Source: CAD feature listing. Evaluate the final solid. Frame: model axes, mm. Give positions to 0.01 mm unless a question says otherwise; leave off trailing zeros. Loops run counter-clockwise (first coordinate to the right, second up) from the corner with the lowest first, then second, coordinate; pieces in that order, holes last. Notation, with made-up numbers: M 4,65.5 L 27,65.5 A21 cw 27,91.5 Z; hole C 5.25,-28.75 d4. An arc over 180 degrees is marked long. Write item = value, one per line.
from build123d import *

# Parameters (mm, degrees)
F0_R     = 2.5
F1_DEPTH = 4.85
F4_DEPTH = 3
F6_DEPTH = 5


with BuildPart() as f1:
    # F0 (on Front) → F1 (new body)
    with BuildSketch(Plane.XZ):
        with BuildLine():
            Line((0, 10.100125), (0, 5))
            Line((0, 5), (-2, 5))
            Line((-2, 5), (-2, -5))
            Line((-2, -5), (0, -5))
            Line((0, -5), (0, -9.588868))
            ThreePointArc((0, -9.588868), (0.776393, -10.563548), (1.9, -10.024758))
            Line((1.9, -10.024758), (1.9, -9.493749))
            Line((1.9, -9.493749), (101.874922, -4.488743))
            Line((101.874922, -4.488743), (106.868668, -4.238743))
            ThreePointArc((106.868668, -4.238743), (111.143668, 0.255629), (106.868668, 4.75))
            Line((106.868668, 4.75), (101.874922, 5))
            Line((101.874922, 5), (1.9, 10.005006))
            Line((1.9, 10.005006), (1.9, 10.71228))
            ThreePointArc((1.9, 10.71228), (0.845568, 11.433139), (0, 10.47581))
            Line((0, 10.47581), (0, 10.100125))
        make_face()
        Polygon((13.94009, -6.988611), (1.9, -7.59137), (1.9, 0.047531), (1.9, 6.476616), align=None, mode=Mode.SUBTRACT)
        Polygon((40.412243, -5.663346), (16.82521, -6.844175), (30.799962, 5.351317), align=None, mode=Mode.SUBTRACT)
        Polygon((43.297363, -5.518909), (54.399668, 4.169854), (62.036187, -4.580795), align=None, mode=Mode.SUBTRACT)
        Polygon((64.921308, -4.436358), (73.677236, 3.204768), (79.699843, -3.696506), align=None, mode=Mode.SUBTRACT)
        Polygon((89.5515, 2.52749), (96.364107, -2.862249), (82.584964, -3.552069), align=None, mode=Mode.SUBTRACT)
        with Locations((106.643668, 0.255629)):
            Circle(F0_R, mode=Mode.SUBTRACT)
        Polygon((15.278104, -5.623766), (3.363279, 8.029371), (29.427927, 6.724507), align=None, mode=Mode.SUBTRACT)
        Polygon((41.750257, -4.298501), (32.254169, 6.583018), (53.027633, 5.543044), align=None, mode=Mode.SUBTRACT)
        Polygon((72.305201, 4.577958), (63.374202, -3.21595), (55.853875, 5.401555), align=None, mode=Mode.SUBTRACT)
        Polygon((88.052204, 3.789622), (81.037857, -2.331661), (75.131443, 4.436469), align=None, mode=Mode.SUBTRACT)
        Polygon((91.211182, 3.631475), (97.850325, 3.299102), (97.850325, -1.621029), align=None, mode=Mode.SUBTRACT)
    extrude(amount=F1_DEPTH)

    # F3 (on offset) → F4 (cut)
    with BuildSketch(Plane.XY.offset(10)):
        Polygon((36, 0), (36, -2.5), (36, -5), (40, -5), (40, -2.5), (40, 0), align=None)
        Polygon((76, 0), (76, -2.5), (76, -5), (80, -5), (80, -2.5), (80, 0), align=None)
    extrude(amount=-F4_DEPTH, mode=Mode.SUBTRACT)

    # F5 (on offset) → F6 (cut)
    with BuildSketch(Plane.XY.offset(10)):
        Polygon((76, 0), (76, -2.5), (76, -5), (80, -5), (80, -2.5), (80, 0), align=None)
    extrude(amount=-F6_DEPTH, mode=Mode.SUBTRACT)


solid = f1.part
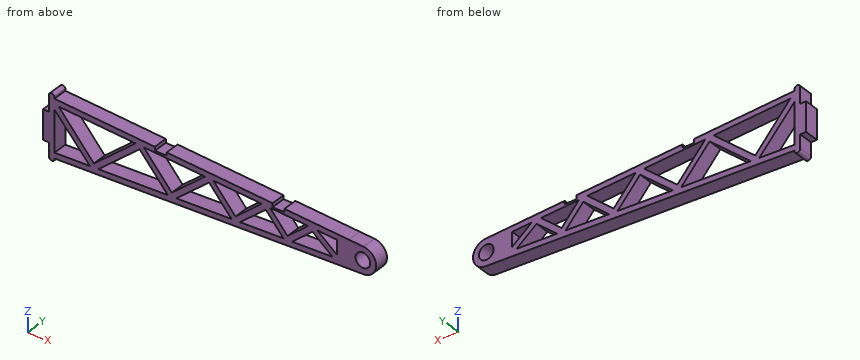
1. Cut plane A-A, the plane x = 67. Return the cut outline in (y, z).
Derived:
outline = M -4.85,-6.23 L 0,-6.23 L 0,-4.33 L -4.85,-4.33 Z; M -4.85,-2.62 L 0,-2.62 L 0,-0.05 L -4.85,-0.05 Z; M -4.85,4.84 L 0,4.84 L 0,6.75 L -4.85,6.75 Z
2. Material intervals for probe 1 along Z at (x, y) = (92, -1); probe 2 along Z at (x, y) = (84.5, -4.05); probe 3 along Z at (x, y) = (82, -3.75) (3 decimals), sorted ascending. Write a range as from..to.
Derived:
probe_1 = -4.98..-3.08, 0.59..3.01, 3.59..5.49
probe_2 = -5.36..-3.46, -1.88..0.69, 3.97..5.87
probe_3 = -5.484..-1.492, 4.093..5.995
3. First-contact query: pin 1 Ø2 at (x, y) = (38.5, -1) entering from +Z; pin 2 Ø2.5 at (y, z) = (-2, -6.5) entering from -X; pin 3 Ø1 at (x, y) = (-1, -2) entering from +Z. Flat tips, straight axial feed; report the tip coordinate or a pass-through.
Derived:
pin_1 = 7
pin_2 = 0
pin_3 = 5
4. Cut plane B-B, the plane x = 9. Return the cut outline in (y, z), then the cut area to 3 significant figures.
Derived:
outline = M -4.85,-9.14 L 0,-9.14 L 0,-7.24 L -4.85,-7.24 Z; M -4.85,-1.46 L 0,-1.46 L 0,1.57 L -4.85,1.57 Z; M -4.85,7.75 L 0,7.75 L 0,9.65 L -4.85,9.65 Z
area = 33.2 mm²
5. Cut plane C-C, the plane y = -1.3. Count the separate pieces of the cut face and the enclosed holes in it, then the cut area to 3 significant figures.
Derived:
separate_pieces = 1
enclosed_holes = 11
area = 754 mm²
